Build history of the part. All positions in model axes, mm. A direction names the side the tool comes from. Round coordinates to 2 decimals unless told otherwise and drop trailing zeros. Write each loop counter-clockwise with the first axis right and the second up, starting at its lowest first coordinate (ties: lowest second). Pieces come first, ordered by that corner, then holes. Notation, with made-up numbers: (77.25, -25) -> (103.25, -25) arc R18 ccw to (103.25, 10) -> close; hole circle Ø1 at (65, 72.5). An arc over 180 degrees is marked (long way). Answer as CSV lines item,"result".
from build123d import *

# Parameters (mm, degrees)
CROQUIS2_W              = 66.675
CROQUIS2_H              = 66.675
SALIENTE_EXTRUIR2_DEPTH = 88.9
CORTAR_EXTRUIR1_DEPTH   = 117.01790608
CROQUIS5_OUTSIDE_W      = 94.593
CROQUIS5_OUTSIDE_H      = 94.593
CROQUIS5_OUTSIDE_R      = 33.3375
CORTAR_EXTRUIR2_DEPTH   = 88.9
CROQUIS6_R              = 25.4
CORTAR_EXTRUIR4_DEPTH   = 19.05
CORTAR_EXTRUIR5_DEPTH   = 31.75
CORTAR_EXTRUIR6_START   = -50.8
CORTAR_EXTRUIR6_DEPTH   = 50.8
CROQUIS9_R              = 3.175
CORTAR_EXTRUIR7_DEPTH   = 60.325


with BuildPart() as part:
    # Croquis2 → Saliente-Extruir2 (new body)
    with BuildSketch(Plane(origin=(0, 0, 0), x_dir=(1, 0, 0), z_dir=(0, 1, 0))):
        Rectangle(CROQUIS2_W, CROQUIS2_H)
    extrude(amount=SALIENTE_EXTRUIR2_DEPTH)

    # Croquis4 → Cortar-Extruir1 (cut, through all)
    with BuildSketch(Plane.ZY.offset(33.3375)):
        Polygon((33.3375, 31.157756203), (0, 88.9), (33.3375, 88.9), align=None)
    extrude(amount=-CORTAR_EXTRUIR1_DEPTH, mode=Mode.SUBTRACT)

    # Croquis5 outside → Cortar-Extruir2 (cut)
    with BuildSketch(Plane.XZ):
        with Locations((-0.0005, 0.0005)):
            Rectangle(CROQUIS5_OUTSIDE_W, CROQUIS5_OUTSIDE_H)
        with Locations(Location((0, 0, 0), (0, 0, 270))):
            Circle(CROQUIS5_OUTSIDE_R, mode=Mode.SUBTRACT)
    extrude(amount=-CORTAR_EXTRUIR2_DEPTH, mode=Mode.SUBTRACT)

    # Croquis6 → Cortar-Extruir4 (cut)
    with BuildSketch(Plane(origin=(0, 88.9, 0), x_dir=(1, 0, 0), z_dir=(0, 1, 0))):
        Circle(CROQUIS6_R)
    extrude(amount=-CORTAR_EXTRUIR4_DEPTH, mode=Mode.SUBTRACT)

    # Croquis7 → Cortar-Extruir5 (cut)
    with BuildSketch(Plane(origin=(0, 69.85, 0), x_dir=(1, 0, 0), z_dir=(0, 1, 0))):
        with BuildLine():
            Line((-9.525, 9.525), (-9.525, -31.947821229))
            Line((-9.525, -31.947821229), (9.525, -31.947821229))
            Line((9.525, -31.947821229), (9.525, 9.525))
            ThreePointArc((9.525, 9.525), (0, 19.05), (-9.525, 9.525))
        make_face()
    extrude(amount=-CORTAR_EXTRUIR5_DEPTH, mode=Mode.SUBTRACT)

    # Croquis8 → Cortar-Extruir6 (cut)
    with BuildSketch(Plane(origin=(0, 88.9, 0), x_dir=(1, 0, 0), z_dir=(0, 1, 0)).offset(CORTAR_EXTRUIR6_START)):
        with BuildLine():
            Line((-30.1752, 14.172022128), (-30.1752, -14.172022128))
            ThreePointArc((-30.1752, -14.172022128), (-33.3375, 0), (-30.1752, 14.172022128))
        make_face()
        with BuildLine():
            Line((30.1498, 14.225978568), (30.1498, -14.225978568))
            ThreePointArc((30.1498, -14.225978568), (33.3375, 0), (30.1498, 14.225978568))
        make_face()
    extrude(amount=CORTAR_EXTRUIR6_DEPTH, mode=Mode.SUBTRACT)

    # Croquis9 → Cortar-Extruir7 (cut)
    with BuildSketch(Plane.ZY.offset(30.1752)):
        with Locations((7.9248, 57.15)):
            Circle(CROQUIS9_R)
    extrude(amount=-CORTAR_EXTRUIR7_DEPTH, mode=Mode.SUBTRACT)


solid = part.part
1. Cut at A-A, the plane x = 0. Write the cut outline in (y, z).
Results found:
outline,"(0, -33.34) -> (88.9, -33.34) -> (88.9, -25.4) -> (69.85, -25.4) -> (69.85, -19.05) -> (38.1, -19.05) -> (38.1, 29.33) -> (31.16, 33.34) -> (0, 33.34) -> close"
2. Mould opens along X. For faces 5 (the cylindrical face through (0.72, 79.51, -25.39)), 6 (the flat face through (0, 0, 0)), 7 (the flat face through (-30.175, 63, -3)) say: +X half, -X half, draft (parallel to the pull), parting line (faces both ways), or undercut.
Results found:
face 5,"undercut"
face 6,"draft"
face 7,"-X half"
3. Cut at D-D, the plane z = -7. Write the cut outline in (x, y) (3 decimals), then the cut area to 3 significant figures.
Results found:
outline,"(-32.594, 0) -> (32.594, 0) -> (32.594, 38.1) -> (30.15, 38.1) -> (30.15, 88.9) -> (24.416, 88.9) -> (24.416, 69.85) -> (9.525, 69.85) -> (9.525, 38.1) -> (-9.525, 38.1) -> (-9.525, 69.85) -> (-24.416, 69.85) -> (-24.416, 88.9) -> (-30.175, 88.9) -> (-30.175, 38.1) -> (-32.594, 38.1) -> close"
area,"4,010 mm2"
4. Cut at C-C, the plane z = 9. Write the cut outline in (x, y) (3 decimals), then the cut area to 3 significant figures.
Results found:
outline,"(-32.1, 0) -> (32.1, 0) -> (32.1, 38.1) -> (30.15, 38.1) -> (30.15, 54.163) -> (9.525, 54.163) -> (9.525, 38.1) -> (-9.525, 38.1) -> (-9.525, 54.163) -> (-30.175, 54.163) -> (-30.175, 38.1) -> (-32.1, 38.1) -> close; (-30.175, 60.137) -> (-9.525, 60.137) -> (-9.525, 69.85) -> (-23.752, 69.85) -> (-23.752, 73.312) -> (-30.175, 73.312) -> close; (9.525, 60.137) -> (30.15, 60.137) -> (30.15, 73.312) -> (23.752, 73.312) -> (23.752, 69.85) -> (9.525, 69.85) -> close"
area,"3,550 mm2"
5. Cut at B-B, the plane y = 57.15. Count the separate pieces of the cut face and the enclosed holes in it, then the cut area to 3 significant figures.
Results found:
separate pieces,"3"
enclosed holes,"0"
area,"1,850 mm2"
6. Drop flat-ended pins along their axis: pin 1 Ø1 at (x, z) = (32, 6.5) entering from +Y; pin 2 Ø4 at (y, z) = (57.15, 7.92) entering from -X; pin 3 Ø6 at (x, z) = (-10, 23.5) entering from +Y; pin 4 Ø1.5 at (x, z) = (-11, -14.5) entering from -Y. Give the stop position or say it passes through.
Results found:
pin 1,"stops at y = 38.1"
pin 2,"passes through"
pin 3,"stops at y = 53.39"
pin 4,"stops at y = 0"
7. Which spindle directions (+Z, -Z, +X, -X, +Y, -Y) get a long thin tool onto all of the face, cutting with end or side? Do faces 1 (the flat face through (9.525, 51, 6)), 2 (the cylindrical face through (19.69, 54.05, 7.24)), 3 (the flat face through (-31, 38.1, 0)), 4 (the flat face through (31, 38.1, 0)). Say none if no direction does.
Results found:
face 1,"+Z, +Y"
face 2,"+X, -X"
face 3,"+Z, -Z, -X, +Y"
face 4,"+Z, -Z, +X, +Y"
8. Probe line 1 along X through (y, z) = (57.5, -2) (3 decimals); line 2 along X through (y, z) = (82.75, 0); line 3 along Y through (x, z) = (-24, 8). List the from-to ranges inside material, lowest first.
Results found:
line 1,"x = -30.175 to -9.525, 9.525 to 30.15"
line 2,"x = -30.18 to -25.4, 25.4 to 30.15"
line 3,"y = 0 to 53.98, 60.32 to 69.85"
